Check sheet for the drawn part. Datum: minimum x, y, z corner. Units: mm. A direction names the side the tool comes from. Round coordinates to 2 decimals unless told otherwise and drop trailing zeros. Write each loop counter-clockwise with the first axis right and the second up, starting at its lowest first coordinate (ties: lowest second). Pieces come first, ordered by that corner, then holes. Notation, with made-up numbers: M 13.25,43.25 L 23.25,43.25 A15 cw 23.25,53.25 Z; hole C 25.25,-20.75 d4. An arc over 180 degrees is marked long. Answer as CSV lines item,"result". Start each with the question number.
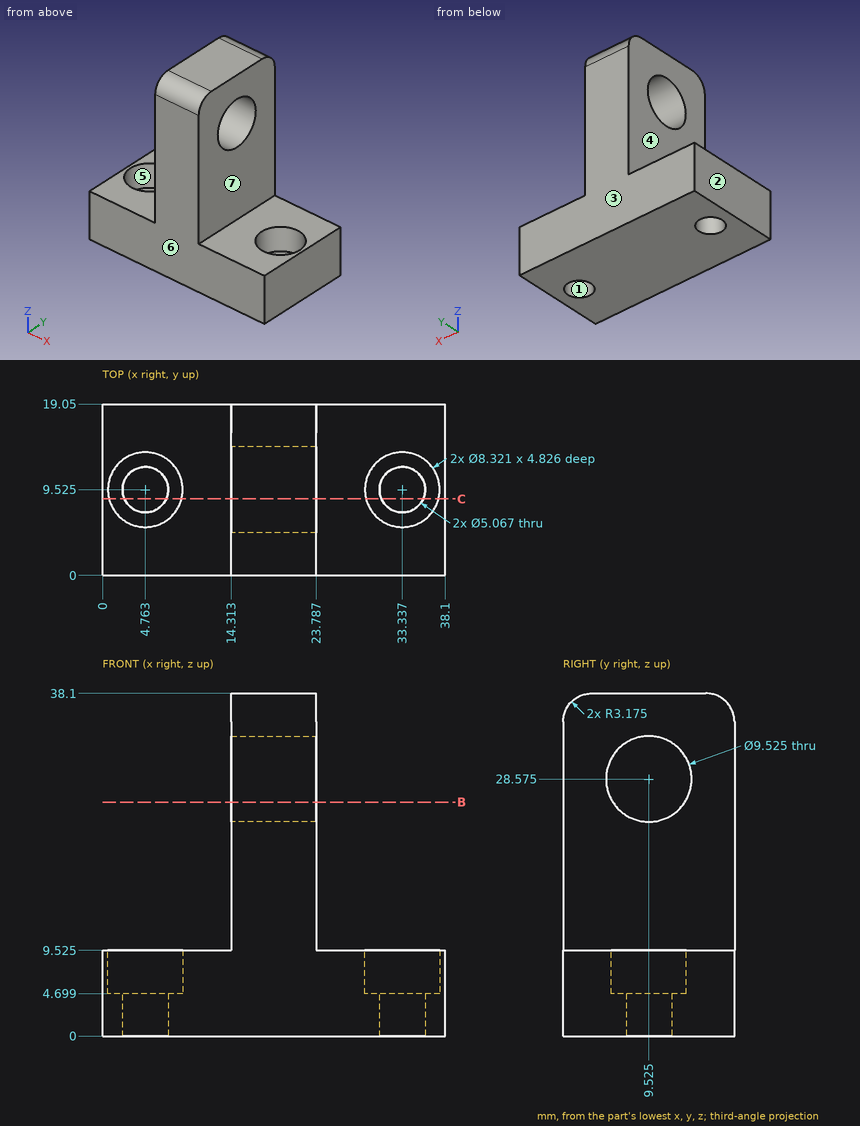
1) Access from +Z, -Z, +X, -X, +Y, -Y to the whole of each face (thin tool, end or side, straight path). Record for the marked faces 4, 5, 6 and 7.
2) Section check B-B, the plane z = 26. Record the cut outline in (x, y).
3) Go/stop test with flat-tipped pins: pin 1 (11 mm diameter, centred on x = 33.34, y = 9.53, fed in from +Z) (1 decimal); pin 2 (4.5 mm diameter, centred on x = 34.5, y = 10, fed in from +Z); pin 3 (5.5 mm diameter, centred on y = 5.5, z = 17, fed in from +X). Record where each tip stops, or that it passes through.
4) Scan lines: line 1 (Z direction, x = 15, y = 9.25); line 2 (Y direction, x = 4.5, z = 6.5); line 3 (Z direction, x = 28, y = 4.25) (1 decimal). Record each from-to range of solid material in increasing order. Write a range as from..to.
5) Section check C-C, the plane y = 8.5. Record the cut outline in (x, z) (1 decimal).
6) Mould release check, pull along X, two halves, no side actions. Record for the marked faces 1, 2 and 3: released by +X, released by -X, zero draft, split by the parting line, or undercut.
Results:
1,face 4,"+Z, -X, +Y, -Y"
1,face 5,"+Z"
1,face 6,"+Z, -Z, +X, -X, -Y"
1,face 7,"+Z, +X, +Y, -Y"
2,outline,"M 14.31,0 L 23.79,0 L 23.79,5.52 L 14.31,5.52 Z; M 14.31,13.53 L 23.79,13.53 L 23.79,19.05 L 14.31,19.05 Z"
3,pin 1,"stops at z = 9.5"
3,pin 2,"stops at z = 4.7"
3,pin 3,"stops at x = 23.79"
4,line 1,"z = 0..23.82, 33.33..38.1"
4,line 2,"y = 0..5.37, 13.68..19.05"
4,line 3,"z = 0..9.5"
5,outline,"M 0,0 L 2.4,0 L 2.4,4.7 L 0.7,4.7 L 0.7,9.5 L 0,9.5 Z; M 7.1,0 L 31,0 L 31,4.7 L 29.3,4.7 L 29.3,9.5 L 23.8,9.5 L 23.8,23.9 L 14.3,23.9 L 14.3,9.5 L 8.8,9.5 L 8.8,4.7 L 7.1,4.7 Z; M 14.3,33.2 L 23.8,33.2 L 23.8,38.1 L 14.3,38.1 Z; M 35.7,0 L 38.1,0 L 38.1,9.5 L 37.4,9.5 L 37.4,4.7 L 35.7,4.7 Z"
6,face 1,"undercut"
6,face 2,"released by -X"
6,face 3,"zero draft"
